```python
from build123d import *

# Parameters (mm, degrees)
SKETCH2_R           = 8
BOSS_EXTRUDE1_DEPTH = 2.85
SKETCH3_W           = 17.15
SKETCH3_H           = 2.85
BOSS_EXTRUDE2_DEPTH = 50
SKETCH4_R           = 1.7
CUT_EXTRUDE1_DEPTH  = 2.85


with BuildPart() as part:
    # Sketch2 → Boss-Extrude1 (new body)
    with BuildSketch(Plane.XY):
        with BuildLine():
            Line((-25, 17.5), (-25, 0))
            ThreePointArc((-25, 0), (-16.787403964, -11.60099689), (-3.116564417, -7.710237508))
            ThreePointArc((-3.116564417, -7.710237508), (0, -6.21763182), (3.116564417, -7.710237508))
            ThreePointArc((3.116564417, -7.710237508), (16.787403964, -11.60099689), (25, 0))
            Line((25, 0), (25, 17.5))
            Line((25, 17.5), (-25, 17.5))
        make_face()
        with Locations((12.7, 0)):
            Circle(SKETCH2_R, mode=Mode.SUBTRACT)
        with Locations((-12.7, 0)):
            Circle(SKETCH2_R, mode=Mode.SUBTRACT)
    extrude(amount=BOSS_EXTRUDE1_DEPTH)

    # Sketch3 → Boss-Extrude2 (add)
    with BuildSketch(Plane.ZY.offset(25)):
        with Locations((-8.575, 16.075)):
            Rectangle(SKETCH3_W, SKETCH3_H)
    extrude(amount=-BOSS_EXTRUDE2_DEPTH)

    # Sketch4 → Cut-Extrude1 (cut)
    with BuildSketch(Plane(origin=(0, 17.5, 0), x_dir=(1, 0, 0), z_dir=(0, 1, 0))):
        with Locations((-7, 12.15)):
            Circle(SKETCH4_R)
        with Locations((7, 12.15)):
            Circle(SKETCH4_R)
    extrude(amount=-CUT_EXTRUDE1_DEPTH, mode=Mode.SUBTRACT)


solid = part.part
```
CAD build for the part. Positions are in the model's coordinates, mm. A direction names the side the tool comes from. Coordinates: 2 decimals unless noted, no trailing zeros. Order: outer loops, then holes, each group sorted by start corner. A loop starts at its lowest first (then second) coordinate and runs counter-clockwise, first axis right, second up.
(1) Which spindle directions (+Z, -Z, +X, -X, +Y, -Y) get a long thin tool onto all of the face, cutting with end or side? Do faces 1 (the face through (0, 17.5, -7)), 2 (the face through (0, 14.65, -9)). Say none if no direction does.
Solution:
face 1: +Z, -Z, +X, -X, +Y
face 2: -Z, +X, -X, -Y
(2) Drill centre lines: L1, parallel to X at y = 16.4, z = -12.15; L2, parallel to Y at x = -12.7, z = 1.45; L3, parallel to Z at x = -7, y = 15.9. Where is each one in solid material? Low to high.
Solution:
L1: x = -25 to -8.7, -5.3 to 5.3, 8.7 to 25
L2: y = -12.3 to -8, 8 to 17.5
L3: z = -17.15 to -13.85, -10.45 to 2.85
(3) Saw through at D-D, the plane x = -7. Write the cut outline in (y, z).
Solution:
outline: (-10.9, 0) - (-5.61, 0) - (-5.61, 2.85) - (-10.9, 2.85) - close; (5.61, 0) - (14.65, 0) - (14.65, -10.45) - (17.5, -10.45) - (17.5, 2.85) - (5.61, 2.85) - close; (14.65, -17.15) - (17.5, -17.15) - (17.5, -13.85) - (14.65, -13.85) - close
(4) Pin check, flat tips, straight feed: pin 1 Ø5.5 at (x, z) = (7, -12.15) entering from -Y; pin 2 Ø4 at (x, z) = (9, -2.5) entering from -Y; pin 3 Ø13.5 at (x, y) = (5, 0.5) entering from -Z. Stop position of each tip, or through.
Solution:
pin 1: stops at y = 14.65
pin 2: stops at y = 14.65
pin 3: stops at z = 0
(5) Saw through at A-A, the plane x = -12.7. Write the cut outline in (y, z), and give its area (3 significant figures).
Solution:
outline: (-12.3, 0) - (-8, 0) - (-8, 2.85) - (-12.3, 2.85) - close; (8, 0) - (14.65, 0) - (14.65, -17.15) - (17.5, -17.15) - (17.5, 2.85) - (8, 2.85) - close
area: 88.2 mm2
(6) Saw through at B-B, the plane z = -12.15. Write the cut outline in (x, y).
Solution:
outline: (-25, 14.65) - (-8.7, 14.65) - (-8.7, 17.5) - (-25, 17.5) - close; (-5.3, 14.65) - (5.3, 14.65) - (5.3, 17.5) - (-5.3, 17.5) - close; (8.7, 14.65) - (25, 14.65) - (25, 17.5) - (8.7, 17.5) - close
(7) Mould opens along Z. For faces 3 (the face through (0, 6, 2.85)), 4 (the face through (0, 16, -17.15)), 5 (the face through (-7.221, 16.095, -13.836)), 6 (the face through (6.779, 16.095, -13.836)) say: released by +Z, released by -Z, zero draft, split by the parting line, or undercut.
Solution:
face 3: released by +Z
face 4: released by -Z
face 5: undercut
face 6: undercut
(8) Saw through at C-C, the plane y = -3.5. Write the cut outline in (x, z).
Solution:
outline: (-24.49, 0) - (-19.89, 0) - (-19.89, 2.85) - (-24.49, 2.85) - close; (-5.51, 0) - (5.51, 0) - (5.51, 2.85) - (-5.51, 2.85) - close; (19.89, 0) - (24.49, 0) - (24.49, 2.85) - (19.89, 2.85) - close
